```python
from build123d import *

# Parameters (mm, degrees)
F0_R     = 3
F1_DEPTH = 1.5


with BuildPart() as f1:
    # F0 (on Front) → F1 (new body)
    with BuildSketch(Plane.XZ):
        with BuildLine():
            Line((4, 3.826665), (6.973982, 34.397026))
            ThreePointArc((6.973982, 34.397026), (0, 42), (-6.973982, 34.397026))
            Line((-6.973982, 34.397026), (-4, 3.826665))
            Line((-4, 3.826665), (-4, 0))
            Line((-4, 0), (-4, -3.826665))
            Line((-4, -3.826665), (-6.973982, -34.397026))
            ThreePointArc((-6.973982, -34.397026), (0, -42), (6.973982, -34.397026))
            Line((6.973982, -34.397026), (4, -3.826665))
            Line((4, -3.826665), (4, 0))
            Line((4, 0), (4, 3.826665))
        make_face()
        with Locations((0, -35)):
            Circle(F0_R, mode=Mode.SUBTRACT)
        with Locations((0, 35)):
            Circle(F0_R, mode=Mode.SUBTRACT)
    extrude(amount=F1_DEPTH)


solid = f1.part
```
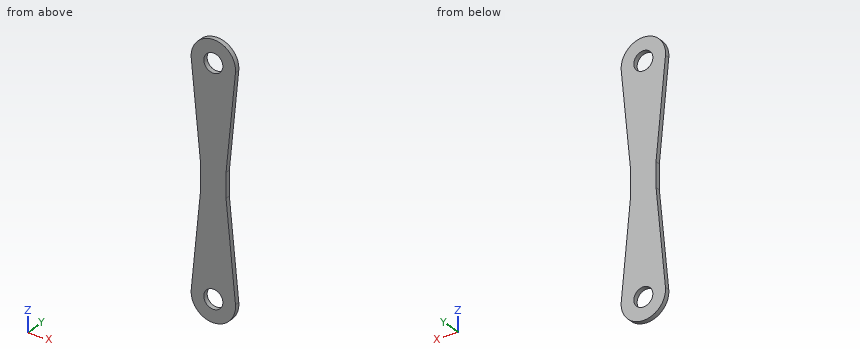
Verification items for the finished model (mm, model axes). Give positions to 0.01 mm unless a question says otherwise; leave off trailing zeros. Loops run counter-clockwise (first coordinate to the right, second up) from the corner with the lowest first, then second, coordinate; pieces in that order, holes last. Notation, with made-up numbers: M -18.75,81.5 L 31.25,81.5 A12 ccw 31.25,100.5 Z; hole C -11,56.5 d9. An arc over 180 degrees is marked long. Return JSON: item names as keys, results as strings.
1) Material ranges on L1, parallel to Z at x = 0, y = -0.4; L2, parallel to Z at x = 1.75, y = -0.25; L3, parallel to X at y = -1.3, z = -4, recorded low to high. Write a range as [from, to].
Findings:
{"L1": "z = [-42, -38], [-32, 32], [38, 42]", "L2": "z = [-41.78, -37.44], [-32.56, 32.56], [37.44, 41.78]", "L3": "x = [-4.02, 4.02]"}
2) Section check A-A, the plane y = -0.25. Enter the section's corners in (x, z), and give its area (3 significant figures).
Findings:
{"outline": "M -6.97,-34.4 A7 ccw long 6.97,-34.4 L 4,-3.83 L 4,3.83 L 6.97,34.4 A7 ccw long -6.97,34.4 L -4,3.83 L -4,-3.83 Z; hole C 0,-35 d6; hole C 0,35 d6", "area": "846 mm2"}
3) Section check D-D, the plane z = -1. Enter the section's corners in (x, y).
Findings:
{"outline": "M -4,-1.5 L 4,-1.5 L 4,0 L -4,0 Z"}
4) Section check B-B, the plane x = 0. Enter the section's corners in (y, z), and give its area (3 significant figures).
Findings:
{"outline": "M -1.5,-42 L 0,-42 L 0,-38 L -1.5,-38 Z; M -1.5,-32 L 0,-32 L 0,32 L -1.5,32 Z; M -1.5,38 L 0,38 L 0,42 L -1.5,42 Z", "area": "108 mm2"}
5) Gauge pin test, flat end, axial feed: P1, Ø3.5, axis at x = 0, z = -35, coming from the +Y side. Record the tip position at first contact, or that the pin passes through.
Findings:
{"P1": "passes through"}
6) Section check C-C, the plane x = 5.5. Enter the section's corners in (y, z), and give its area (3 significant figures).
Findings:
{"outline": "M -1.5,-39.33 L 0,-39.33 L 0,-19.25 L -1.5,-19.25 Z; M -1.5,19.25 L 0,19.25 L 0,39.33 L -1.5,39.33 Z", "area": "60.3 mm2"}
